Could you check a few things on this model? Use its own coordinates, in mm. A direction names the side the tool comes from. Round coordinates to 2 decimals unless told otherwise and drop trailing zeros. Write each loop counter-clockwise with the first axis right and the second up, starting at its lowest first coordinate (ties: lowest second). Pieces come first, ordered by that corner, then holes. Notation, with made-up numbers: (86.5, 6.5) -> (124.5, 6.5) arc R30 cw to (124.5, 39.5) -> close; hole circle Ø1 at (19, 55). An arc over 180 degrees is marked (long way). Return JSON: item names as keys, results as strings.
Autodesk Inventor part; units mm, degrees
ref_plane "YZ Plane" through (0, 0, 0) normal (1, 0, 0) x (0, 1, 0)
ref_plane "XZ Plane" through (0, 0, 0) normal (0, 1, 0) x (-1, 0, 0)
ref_plane "XY Plane" through (0, 0, 0) normal (0, 0, 1) x (1, 0, 0)
sketch "Sketch1" plane through (0, 0, 0) normal (0, 1, 0) x (-1, 0, 0)
  line L0 (31.75, 37) -> (-31.75, 37)
  line L1 (-31.75, 37) -> (-31.75, -37)
  line L2 (-31.75, -37) -> (31.75, -37)
  line L3 (31.75, -37) -> (31.75, 37)
  point P0 (0, 0)
  point P1 (31.75, 0)
  point P2 (0, 37)
  dimension "d0" = 74
  dimension "d1" = 63.5
extrude "Extrusion1" add sketch "Sketch1" along normal blind 0.96
sketch "Sketch2" plane through (0, 0.96, 0) normal (0, 1, 0) x (1, 0, 0)
  line L0 (31.75, -37) -> (31.75, 37)
  line L1 (31.75, 37) -> (-31.75, 37)
  line L2 (-31.75, 37) -> (-31.75, -37)
  line L3 (-31.75, -37) -> (31.75, -37)
  line L4 (-31.75, 0) -> (31.75, 0)
  line L5 (0, -37) -> (0, 37)
  circle A0 centre (-16, -16) radius 4.25
  circle A1 centre (-16, 16) radius 4.25
  circle A2 centre (16, 16) radius 4.25
  circle A3 centre (16, -16) radius 4.25
  point P0 (0, 0)
  dimension "d13" = 8.5
  dimension "d14" = 32
  dimension "d15" = 32
extrude "Extrusion2" add sketch "Sketch2" along normal blind 1.92
sketch "Sketch3" plane through (0, 2.88, 0) normal (0, 1, 0) x (1, 0, 0)
  line L0 (-31.75, 37) -> (-31.75, -37)
  line L1 (-31.75, -37) -> (31.75, -37)
  line L2 (31.75, -37) -> (31.75, 37)
  line L3 (31.75, 37) -> (-31.75, 37)
  point P0 (0, 0)
extrude "Extrusion3" add sketch "Sketch3" along normal blind 0.64
fillet "Fillet1" radius 8 4 edges at (31.75, 1.76, 37) (-31.75, 1.76, 37) (-31.75, 1.76, -37) (31.75, 1.76, -37)
ref_plane "Arbeitsebene2" through (29.4069, 3.52, -34.6569) normal (-0.7625, 0, -0.647) x (0, -1, 0)
sketch "Skizze7" plane through (0, 3.52, 0) normal (0, 1, 0) x (1, 0, 0)
  line L0 (-23.75, -37) -> (23.75, -37)
  arc A0 (23.75, -37) -> (31.75, -29) centre (23.75, -29) ccw
  line L1 (31.75, -29) -> (31.75, 29)
  arc A1 (31.75, 29) -> (23.75, 37) centre (23.75, 29) ccw
  line L2 (23.75, 37) -> (-23.75, 37)
  arc A2 (-23.75, 37) -> (-31.75, 29) centre (-23.75, 29) ccw
  line L3 (-31.75, 29) -> (-31.75, -29)
  arc A3 (-31.75, -29) -> (-23.75, -37) centre (-23.75, -29) ccw
  line L4 (23.75, -37) -> (-27, -37)
  line L5 (-31.75, -29) -> (-31.75, 29)
  line L6 (-23.75, 37) -> (23.75, 37)
  line L7 (31.75, 29) -> (31.75, -29)
  arc A4 (23.75, -37) -> (31.75, -29) centre (23.75, -29) ccw
  arc A5 (-32.385, -29) -> (-27, -37) centre (-23.75, -29) ccw
  arc A6 (-23.75, 37) -> (-31.75, 29) centre (-23.75, 29) ccw
  arc A7 (31.75, 29) -> (23.75, 37) centre (23.75, 29) ccw
  point P0 (0, 0)
extrude "Extrusion4" add sketch "Skizze7" along normal blind 3.2
sketch "Skizze8" plane through (0, 6.72, 0) normal (0, 1, 0) x (1, 0, 0)
  line L0 (25.25, 30.5) -> (-25.25, 30.5)
  line L1 (-25.25, 30.5) -> (-25.25, -30.5)
  line L2 (-25.25, -30.5) -> (25.25, -30.5)
  line L3 (25.25, -30.5) -> (25.25, 30.5)
  line L4 (25.25, 30.5) -> (-25.25, -30.5) construction
  line L5 (-25.25, 30.5) -> (25.25, -30.5) construction
  point P0 (0, 0)
  dimension "d25" = 61
  dimension "d26" = 50.5
extrude "Extrusion5" cut sketch "Skizze8" against normal blind 3.2
chamfer "Fasen3" distance 5 angle 45 8 edges at (31.75, 6.72, 0) (29.4069, 6.72, -34.6569) (0, 6.72, -37) (-29.4069, 6.72, -34.6569) (-31.75, 6.72, 0) (-29.4069, 6.72, 34.6569) (0, 6.72, 37) (29.4069, 6.72, 34.6569)
properties part number "IMU_Base_T-Shirt"
1) Thinking about a two-plate mould opening in Z: for faces 1 (the face through (-29.285, 4.185, -0.406)), 2 (the face through (25.25, 5, 0)), 3 (the face through (0, 1, 37)), 4 (the face through (15.08, 1.91, -20.15)), which applies, pulls with the +Z half, pulls with the -Z half, needs draft (parallel to the pull), parting line crosses it, or undercut?
Return value:
{"face 1": "needs draft", "face 2": "undercut", "face 3": "pulls with the +Z half", "face 4": "undercut"}
2) I want a section at A-A, the plane x = -16. Please give me the cut outline in (y, z).
Return value:
{"outline": "(0, -37) -> (1.72, -37) -> (6.72, -32) -> (6.72, -30.5) -> (3.52, -30.5) -> (3.52, 30.5) -> (6.72, 30.5) -> (6.72, 32) -> (1.72, 37) -> (0, 37) -> close; hole (0.96, -20.25) -> (2.88, -20.25) -> (2.88, -11.75) -> (0.96, -11.75) -> close; hole (0.96, 11.75) -> (2.88, 11.75) -> (2.88, 20.25) -> (0.96, 20.25) -> close"}
3) For faces 5 (the face through (-16, 0.96, -16)), 6 (the face through (0.332, 4.185, -34.535)), 7 (the face through (-25.25, 5, 0)), which set-ups out of +Z, -Z, +X, -X, +Y, -Y let a thin tool reach every point of the face, with its end or its side?
Return value:
{"face 5": "none", "face 6": "-Z, +X, -X, +Y", "face 7": "+Y"}
4) Will these pins go through, and if not, where does the flat tip stop? pin 1 Ø13.5 at (x, z) = (-16, -16) entering from +Y; pin 2 Ø1 at (y, z) = (4.5, 0) entering from -X; pin 3 Ø2.5 at (y, z) = (5, -12.5) entering from -X.
Return value:
{"pin 1": "y = 3.52", "pin 2": "x = -29.47", "pin 3": "x = -29.72"}
5) I want a section at C-C, the plane z = 16. Please give me the cut outline in (x, y), and give its area (3 significant figures).
Return value:
{"outline": "(-31.75, 0) -> (31.75, 0) -> (31.75, 1.72) -> (26.75, 6.72) -> (25.25, 6.72) -> (25.25, 3.52) -> (-25.25, 3.52) -> (-25.25, 6.72) -> (-26.75, 6.72) -> (-31.75, 1.72) -> close; hole (-20.25, 0.96) -> (-11.75, 0.96) -> (-11.75, 2.88) -> (-20.25, 2.88) -> close; hole (11.75, 0.96) -> (20.25, 0.96) -> (20.25, 2.88) -> (11.75, 2.88) -> close", "area": "207 mm²"}
6) I want a section at D-D, the plane x = 10. Please give me the cut outline in (y, z), and give its area (3 significant figures).
Return value:
{"outline": "(0, -37) -> (1.72, -37) -> (6.72, -32) -> (6.72, -30.5) -> (3.52, -30.5) -> (3.52, 30.5) -> (6.72, 30.5) -> (6.72, 32) -> (1.72, 37) -> (0, 37) -> close", "area": "277 mm²"}
7) If I drill on probe 1 along X at (y, z) = (1.6, 16); probe 2 along X at (y, z) = (1.95, 16); probe 3 along Z at (x, y) = (16, 2.25), over which ranges is the centre line in solid material (lowest first)? Write a range as [from, to].
Return value:
{"probe 1": "[-31.75, -20.25], [-11.75, 11.75], [20.25, 31.75]", "probe 2": "[-31.52, -20.25], [-11.75, 11.75], [20.25, 31.52]", "probe 3": "[-36.47, -20.25], [-11.75, 11.75], [20.25, 36.47]"}
8) I want a section at B-B, the plane y = 5.75. Please give me the cut outline in (x, z), and give its area (3 significant figures).
Return value:
{"outline": "(-27.72, -29) arc R3.97 ccw to (-23.75, -32.97) -> (23.75, -32.97) arc R3.97 ccw to (27.72, -29) -> (27.72, 29) arc R3.97 ccw to (23.75, 32.97) -> (-23.75, 32.97) arc R3.97 ccw to (-27.72, 29) -> close; hole (-25.25, -30.5) -> (25.25, -30.5) -> (25.25, 30.5) -> (-25.25, 30.5) -> close", "area": "562 mm²"}
